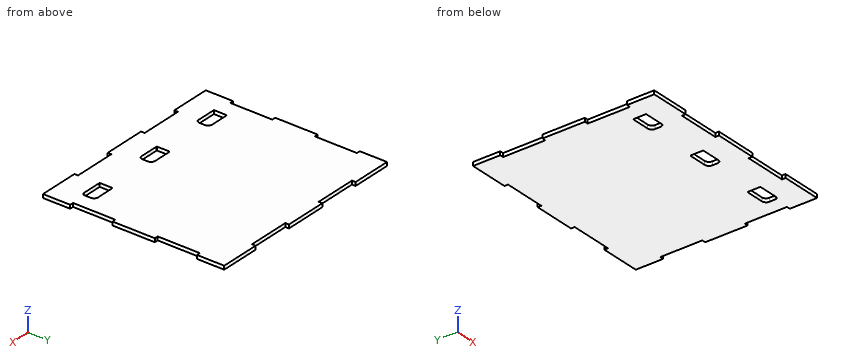
from build123d import *

# Parameters (mm, degrees)
BOSS_EXTRUDE1_DEPTH = 3
CUT_EXTRUDE1_DEPTH  = 114.772799913


with BuildPart() as part:
    # Model → Boss-Extrude1 (new body)
    with BuildSketch(Plane.XY):
        Polygon((85.5, 75), (82.5, 75), (52.5, 75), (52.5, 72), (17.5, 72), (17.5, 75), (-17.5, 75), (-17.5, 72), (-52.5, 72), (-52.5, 75), (-82.5, 75), (-85.5, 75), (-85.5, 72), (-85.5, 52.5), (-82.5, 52.5), (-82.5, 17.5), (-85.5, 17.5), (-85.5, -17.5), (-82.5, -17.5), (-82.5, -52.5), (-85.5, -52.5), (-85.5, -72), (-85.5, -75), (-82.5, -75), (-52.5, -75), (-52.5, -72), (-17.5, -72), (-17.5, -75), (17.5, -75), (17.5, -72), (52.5, -72), (52.5, -75), (82.5, -75), (85.5, -75), (85.5, -72), (85.5, -52.5), (82.5, -52.5), (82.5, -17.5), (85.5, -17.5), (85.5, 17.5), (82.5, 17.5), (82.5, 52.5), (85.5, 52.5), (85.5, 72), align=None)
    extrude(amount=BOSS_EXTRUDE1_DEPTH)

    # Sketch1 → Cut-Extrude1 (cut, through all)
    with BuildSketch(Plane.XY.offset(3)):
        with BuildLine():
            Line((-52.4625, -55), (-68.5375, -55))
            ThreePointArc((-68.5375, -55), (-68.608210678, -54.970710678), (-68.6375, -54.9))
            Line((-68.6375, -54.9), (-68.6375, -45.2))
            ThreePointArc((-68.6375, -45.2), (-68.344606781, -44.492893219), (-67.6375, -44.2))
            Line((-67.6375, -44.2), (-53.3625, -44.2))
            ThreePointArc((-53.3625, -44.2), (-50.869948596, -45.232448596), (-49.8375, -47.725))
            Line((-49.8375, -47.725), (-49.8375, -52.375))
            ThreePointArc((-49.8375, -52.375), (-50.606344699, -54.231155301), (-52.4625, -55))
        make_face()
        with BuildLine():
            Line((7.5375, -55), (-8.5375, -55))
            ThreePointArc((-8.5375, -55), (-8.608210678, -54.970710678), (-8.6375, -54.9))
            Line((-8.6375, -54.9), (-8.6375, -45.2))
            ThreePointArc((-8.6375, -45.2), (-8.344606781, -44.492893219), (-7.6375, -44.2))
            Line((-7.6375, -44.2), (6.6375, -44.2))
            ThreePointArc((6.6375, -44.2), (9.130051404, -45.232448596), (10.1625, -47.725))
            Line((10.1625, -47.725), (10.1625, -52.375))
            ThreePointArc((10.1625, -52.375), (9.393655301, -54.231155301), (7.5375, -55))
        make_face()
        with BuildLine():
            Line((67.5375, -55), (51.4625, -55))
            ThreePointArc((51.4625, -55), (51.391789322, -54.970710678), (51.3625, -54.9))
            Line((51.3625, -54.9), (51.3625, -45.2))
            ThreePointArc((51.3625, -45.2), (51.655393219, -44.492893219), (52.3625, -44.2))
            Line((52.3625, -44.2), (66.6375, -44.2))
            ThreePointArc((66.6375, -44.2), (69.130051404, -45.232448596), (70.1625, -47.725))
            Line((70.1625, -47.725), (70.1625, -52.375))
            ThreePointArc((70.1625, -52.375), (69.393655301, -54.231155301), (67.5375, -55))
        make_face()
    extrude(amount=-CUT_EXTRUDE1_DEPTH, mode=Mode.SUBTRACT)


solid = part.part
Could you check a few things on this model? Use its own coordinates, in mm. Give positions to 0.01 mm unless a question says otherwise; leave off trailing zeros. Order: outer loops, then holes, each group sorted by start corner. A loop starts at its lowest first (then second) coordinate and runs counter-clockwise, first axis right, second up.
Item 1: If we section it at B-B, the plane z = 0.9: Count the separate pieces of the cut face and the enclosed holes in it, plus the area to 3 significant figures.
Item 2: I'm going to push flat-ended pins straight in: pin 1 (12 mm diameter, centred on x = -57.5, y = -22.5, fed in from -Z); pin 2 (0.9 mm diameter, centred on y = -29.5, z = 1, fed in from +X); pin 3 (0.9 mm diameter, centred on y = -27.5, z = 2, fed in from -X). Where does each tip first touch, or does it pass through?
Item 3: If we section it at A-A, the plane x = 64: Write out the boundary of the cut face in (y, z).
Item 4: I need wall thicknesses on line 1 (X direction, y = -48, z = 0.4); line 2 (Y direction, x = 62, z = 1.75); line 3 (X direction, y = -31, z = 0.1). Which ranges of each line are inside material? Lowest first, please.
Item 5: If we section it at C-C, the plane x = -35.5: Write out the boundary of the cut face in (y, z), plus the area to 3 significant figures.
Item 6: If we section it at D-D, the plane y = 20: Write out the boundary of the cut face in (x, z), plus the area to 3 significant figures.
Values:
1. separate pieces: 1
1. enclosed holes: 3
1. area: 24,200 mm2
2. pin 1: stops at z = 0
2. pin 2: stops at x = 82.5
2. pin 3: stops at x = -82.5
3. outline: (-75, 0) - (-55, 0) - (-55, 3) - (-75, 3) - close; (-44.2, 0) - (75, 0) - (75, 3) - (-44.2, 3) - close
4. line 1: x = -82.5 to -68.64, -49.84 to -8.64, 10.16 to 51.36, 70.16 to 82.5
4. line 2: y = -75 to -55, -44.2 to 75
4. line 3: x = -82.5 to 82.5
5. outline: (-72, 0) - (72, 0) - (72, 3) - (-72, 3) - close
5. area: 432 mm2
6. outline: (-82.5, 0) - (82.5, 0) - (82.5, 3) - (-82.5, 3) - close
6. area: 495 mm2
